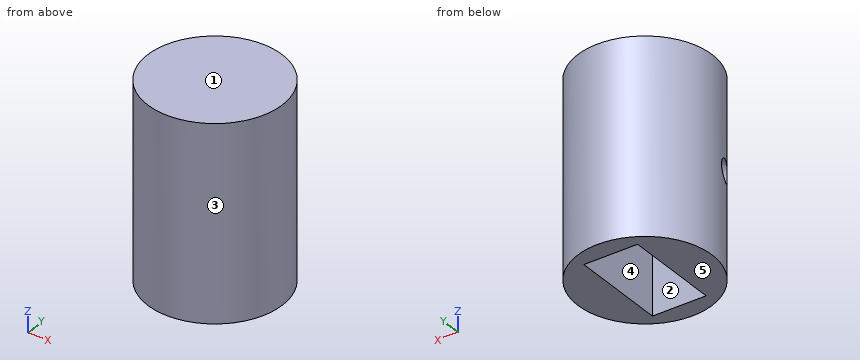
```python
from build123d import *

# Parameters (mm, degrees)
F0_R      = 12.5
F1_DEPTH  = 36
F2_W      = 10
F2_H      = 16
F3_DEPTH  = 32
F4_W      = 10
F4_H      = 2
F5_DEPTH  = 14
F7_D      = 4
F7_DEPTH  = 7.501
F9_W      = 4
F9_H      = 1.1
F10_DEPTH = 8
F8_R      = 3
F8_R_2    = 2.5
F11_DEPTH = 1.5


with BuildPart() as f1:
    # F0 (on Top) → F1 (new body)
    with BuildSketch(Plane.XY):
        Circle(F0_R)
    extrude(amount=F1_DEPTH)

    # F2 (on face) → F3 (cut)
    with BuildSketch(Plane(origin=(0, 0, 0), x_dir=(1, 0, 0), z_dir=(0, 0, -1))):
        with Locations((0, -1)):
            Rectangle(F2_W, F2_H)
    extrude(amount=-F3_DEPTH, mode=Mode.SUBTRACT)

    # F4 (on face) → F5 (cut)
    with BuildSketch(Plane(origin=(0, 0, 0), x_dir=(1, 0, 0), z_dir=(0, 0, -1))):
        with Locations((0, 8)):
            Rectangle(F4_W, F4_H)
    extrude(amount=-F5_DEPTH, mode=Mode.SUBTRACT)

    # F7 (through all, one way)
    with BuildSketch(Plane.YZ.offset(-5)):
        with Locations((-5, 18)):
            Circle(F7_D / 2)
    extrude(amount=-F7_DEPTH, mode=Mode.SUBTRACT)

    # F9 (on face) → F10 (cut)
    with BuildSketch(Plane(origin=(0, 0, 14), x_dir=(1, 0, 0), z_dir=(0, 0, -1))):
        with Locations((-3, 7.55)):
            Rectangle(F9_W, F9_H)
    extrude(amount=-F10_DEPTH, mode=Mode.SUBTRACT)

    # F8 (on face) → F11 (join)
    with BuildSketch(Plane.YZ.offset(-5)):
        with Locations((-5, 18)):
            Circle(F8_R)
        with Locations((-5, 18)):
            Circle(F8_R_2, mode=Mode.SUBTRACT)
    extrude(amount=F11_DEPTH)


solid = f1.part
```
Can you work these out from the model? Positions are in its coordinate system, mm. Face numbers are marked on the shaded views. A direction names the side the tool comes from. Coordinates: 2 decimals unless noted, no trailing zeros. Order: outer loops, then holes, each group sorted by start corner. A loop starts at its lowest first (then second) coordinate and runs counter-clockwise, first axis right, second up.
1. For the marked faces 1 and 2, which set-ups out of +Z, -Z, +X, -X, +Y, -Y let a thin tool reach every point of the face, with its end or its side?
2. I need wall thicknesses on line 1 (Z direction, x = -4.55, y = -5); line 2 (Z direction, x = -7.25, y = -5); line 3 (X direction, y = 6, z = 19). Which ranges of each line are inside material? Lowest first, please.
3. If we section it at A-A (z = 21.5): Please give me the cut outline in (x, y), then the cut area to 3 significant figures.
4. If we section it at B-B (x = -4): Please give me the cut outline in (y, z), then the cut area to 3 significant figures.
5. I'm going to push flat-ended pins straight in: pin 1 (3 mm diameter, centred on x = -3.5, z = 19, fed in from +Y); pin 2 (6 mm diameter, centred on x = 0.5, z = 28, fed in from -Y); pin 3 (1 mm diameter, centred on x = -9, z = 24, fed in from +Y); pin 4 (3 mm diameter, centred on y = 2, z = 13, fed in from +X). Where does each tip first touch, or does it pass through?
6. If we section it at C-C (x = 0.5): Please give me the cut outline in (y, z), then the cut area to 3 significant figures.
7. If we section it at D-D (y = -5): Please give me the cut outline in (x, z), then the cut area to 3 significant figures.
8. Thinking about a two-plate mould opening in X: for the marked faces 3, 4 and 5, which applies, +X half, -X half, draft (parallel to the pull), parting line (faces both ways), or undercut?
Entries:
1. face 1: +Z, +X, -X, +Y, -Y
1. face 2: -Z
2. line 1: z = 15 to 15.5, 20.5 to 21, 32 to 36
2. line 2: z = 0 to 16, 20 to 36
2. line 3: x = -10.97 to -5, 5 to 10.97
3. outline: circle Ø25 at (0, 0); hole (-5, -8.1) - (-1, -8.1) - (-1, -7) - (5, -7) - (5, 9) - (-5, 9) - close
3. area: 326 mm2
4. outline: (-11.84, 0) - (-9, 0) - (-9, 14) - (-8.1, 14) - (-8.1, 22) - (-7, 22) - (-7, 32) - (9, 32) - (9, 0) - (11.84, 0) - (11.84, 36) - (-11.84, 36) - close; circle Ø6 at (-5, 18); hole circle Ø5 at (-5, 18)
4. area: 313 mm2
5. pin 1: stops at y = 12.34
5. pin 2: stops at y = -12.5
5. pin 3: stops at y = 9.17
5. pin 4: stops at x = 12.49
6. outline: (-12.49, 0) - (-9, 0) - (-9, 14) - (-7, 14) - (-7, 32) - (9, 32) - (9, 0) - (12.49, 0) - (12.49, 36) - (-12.49, 36) - close
6. area: 359 mm2
7. outline: (-11.46, 0) - (-5, 0) - (-5, 15) - (-3.5, 15) - (-3.5, 15.5) - (-5, 15.5) - (-5, 16) - (-11.46, 16) - close; (-11.46, 20) - (-5, 20) - (-5, 20.5) - (-3.5, 20.5) - (-3.5, 21) - (-5, 21) - (-5, 32) - (5, 32) - (5, 0) - (11.46, 0) - (11.46, 36) - (-11.46, 36) - close
7. area: 481 mm2
8. face 3: parting line
8. face 4: undercut
8. face 5: draft
